```python
from build123d import *

# Parameters (mm, degrees)
CUT_EXTRUDE10_DEPTH = 1.984375


with BuildPart() as part:
    # Sketch22 → Revolve1 (revolve)
    with BuildSketch(Plane(origin=(0, 0, 0), x_dir=(0, 0, -1), z_dir=(1, 0, 0)), mode=Mode.PRIVATE) as revolve1_sk:
        Polygon((-4.239814779, 0), (-4.239814779, 2.54), (-3.795182992, 3.175), (3.849973798, 3.175), (5.285185221, 1.739788577), (4.239814779, 0), align=None)
    revolve(revolve1_sk.sketch.rotate(Axis((0, 0, -4.239814779), (0, 0, -1)), 180), axis=Axis((0, 0, -4.239814779), (0, 0, -1)))

    # Sketch23 → Cut-Extrude10 (cut)
    with BuildSketch(Plane.XY.offset(4.239814779)):
        Polygon((0, 1.833087105), (-1.5875, 0.916543552), (-1.5875, -0.916543552), (0, -1.833087105), (1.5875, -0.916543552), (1.5875, 0.916543552), align=None)
    extrude(amount=-CUT_EXTRUDE10_DEPTH, mode=Mode.SUBTRACT)

    # Cut-Extrude11 cone 1 section (on through the dimple's axis) → Cut-Extrude11 (revolve, cut)
    with BuildSketch(Plane(origin=(0, 0, 4.239814779), x_dir=(0, -1, 0), z_dir=(1, 0, 0))):
        Polygon((0, 0), (1.833087105, 0), (0, 1.833087105), align=None)
    revolve(axis=Axis((0, 0, 4.239814779), (0, 0, -1)), mode=Mode.SUBTRACT)

    # Cut-Extrude12 cone 1 section (on through the dimple's axis) → Cut-Extrude12 (revolve, cut)
    with BuildSketch(Plane(origin=(0, 0, 2.255439779), x_dir=(0, -1, 0), z_dir=(1, 0, 0))):
        Polygon((0, 0), (1.5875, 0), (0, 0.916543552), align=None)
    revolve(axis=Axis((0, 0, 2.255439779), (0, 0, -1)), mode=Mode.SUBTRACT)


solid = part.part
```
Build history of the part. All positions in model axes, mm. A direction names the side the tool comes from. Round coordinates to 2 decimals unless told otherwise and drop trailing zeros. Order: outer loops, then holes, each group sorted by start corner. A loop starts at its lowest first (then second) coordinate and runs counter-clockwise, first axis right, second up. Notation, with made-up numbers: (28, 31) - (53, 31) arc R21 cw to (53, 55) - close; hole circle Ø11 at (18, 6.5). An arc over 180 degrees is marked (long way). Use a Markdown table: item, result.
1) Pull direction Y, two halves, no side cores. Call faces 3 (the face through (0.783, -1.381, 3.262)), 4 (the face through (2, 1, 4.24)), 5 (the face through (2.8, -1.5, -0.1)), 6 (the face through (0.247, 0.055, 1.485)): pulls with the +Y half, pulls with the -Y half, needs draft (parallel to the pull), parting line crosses it, or undercut.
Recorded:
| item | result |
|---|---|
| face 3 | undercut |
| face 4 | needs draft |
| face 5 | parting line crosses it |
| face 6 | undercut |
2) Wall check: L1, parallel to Y at x = -1, z = 0; L2, parallel to Y at x = 0.5, z = 3.25; L3, parallel to Z at x = -1, y = 0.5. Give the ranges that are in metal, low to high.
Recorded:
| item | result |
|---|---|
| L1 | y = -3.01 to 3.01 |
| L2 | y = -3.14 to -1.54, 1.54 to 3.14 |
| L3 | z = -4.91 to 1.98 |
3) Saw through at B-B on z = 0. Write the cut outline in (x, y) (3 decimals).
Recorded:
| item | result |
|---|---|
| outline | circle Ø6.35 at (0, 0) |
4) Saw through at C-C on z = -4.5. Write the cut outline in (x, y), and give its area (3 significant figures).
Recorded:
| item | result |
|---|---|
| outline | circle Ø5.05 at (0, 0); hole circle Ø0.87 at (0, 0) |
| area | 19.4 mm² |
5) Tool access for faces 1 (the face through (0.271, 0.06, -4.407)), 2 (the face through (-0.783, 1.381, 3.262)): list every direction of +Z, -Z, +X, -X, +Y, -Y with a clear straight run to the whole face (end or side of a thin tool).
Recorded:
| item | result |
|---|---|
| face 1 | -Z |
| face 2 | +Z |
6) Flat gauge pins, fed straight in: pin 1 Ø0.6 at (x, y) = (1, -1) entering from +Z; pin 2 Ø0.6 at (x, y) = (-1, 0.5) entering from +Z. Where does each tip first touch, or does it go through?
Recorded:
| item | result |
|---|---|
| pin 1 | stops at z = 4.12 |
| pin 2 | stops at z = 2.16 |
